from build123d import *

# Parameters (mm, degrees)
SKETCH_2_W          = 40
SKETCH_2_H          = 57
CUT_EXTRUDE_1_DEPTH = 4
SKETCH_3_R          = 7
CUT_EXTRUDE_3_DEPTH = 4


with BuildPart() as part:
    # 草圖1 → 旋轉1 (revolve)
    with BuildSketch(Plane.XY):
        Polygon((0, 21), (25, 21), (25, 0), (28.5, 0), (28.5, -2), (12.5, -2), (12.5, -21.7), (8, -21.7), (8, 2.3), (0, 2.3), align=None)
    revolve(axis=Axis((0, 41.921070153, 0), (0, -1, 0)))

    # 草圖2 → 除料-伸長1 (cut)
    with BuildSketch(Plane(origin=(0, 21, 0), x_dir=(1, 0, 0), z_dir=(0, 1, 0))):
        Rectangle(SKETCH_2_W, SKETCH_2_H)
    extrude(amount=-CUT_EXTRUDE_1_DEPTH, mode=Mode.SUBTRACT)

    # 草圖3 → 除料-伸長3 (cut)
    with BuildSketch(Plane(origin=(0, 17, 0), x_dir=(1, 0, 0), z_dir=(0, 1, 0))):
        Circle(SKETCH_3_R)
    extrude(amount=-CUT_EXTRUDE_3_DEPTH, mode=Mode.SUBTRACT)


solid = part.part
Source: CAD feature listing. Evaluate the final solid. Frame: model axes, mm. A direction names the side the tool comes from. Round coordinates to 2 decimals unless told otherwise and drop trailing zeros. Loops run counter-clockwise (first coordinate to the right, second up) from the corner with the lowest first, then second, coordinate; pieces in that order, holes last.
Q1. Section A-A, the plane x = 0. Return loops of the section in (y, z), plus the area to 3 significant figures.
Q2. Ray query, line 1 (X direction, y = 14.7, z = 0); line 2 (Y direction, x = -8.5, z = 22.5). Return the intervals inside material, ascending.
Q3. First-contact query: P1, Ø4, axis at x = -13.5, y = -1, coming from the -Z side; P2, Ø1, axis at x = 13, y = 2.5, coming from the +Z side; P3, Ø15.5, axis at x = -1, z = 2, coming from the +Y side; P4, Ø6, axis at x = -1.5, z = 7, coming from the -Y side. Flat tips, straight axial feed; report the tip coordinate or a pass-through.
Q4. Section D-D, the plane z = 0. Return loops of the section in (x, y), plus the area to 3 significant figures.
Q5. Section B-B, the plane z = 21.5. Return loops of the section in (x, y).
Q6. Access query for faces 1 (the face through (-22, 21, 0)), 2 (the face through (26.327, -1.014, -10.916)), 3 (the face through (-1.73, -9.53, -7.81)), 4 (the face through (6.466, 15.028, 2.681)), 5 (the face through (-5, 17, -6)). Directions: +Z, -Z, +X, -X, +Y, -Y. A direction counts if a zero-diameter tool reaches every point of the face in a straight line with its end or side. Return the directions, or none.
Q7. Mould query, pull axis Z, two halves, no side actions, for faces 6 (the face through (-0.2, -21.7, -8.2)), 7 (the face through (0, 13, 0)), 8 (the face through (11.923, -11.988, 3.755)). Classes: pulls with the +Z half, pulls with the -Z half, needs draft (parallel to the pull), parting line crosses it, or undercut.
Q8. Section C-C, the plane y = 1.5. Return loops of the section in (x, z).
Solutions:
1. outline: (-21.7, -12.5) - (-2, -12.5) - (-2, -28.5) - (0, -28.5) - (0, -25) - (17, -25) - (17, -7) - (13, -7) - (13, 7) - (17, 7) - (17, 25) - (0, 25) - (0, 28.5) - (-2, 28.5) - (-2, 12.5) - (-21.7, 12.5) - (-21.7, 8) - (2.3, 8) - (2.3, -8) - (-21.7, -8) - close
1. area: 1,020 mm2
2. line 1: x = -25 to -7, 7 to 25
2. line 2: y = -2 to 17
3. P1: stops at z = -26.08
3. P2: stops at z = 21.65
3. P3: stops at y = 17
3. P4: stops at y = -21.7
4. outline: (-28.5, -2) - (-12.5, -2) - (-12.5, -21.7) - (-8, -21.7) - (-8, 2.3) - (8, 2.3) - (8, -21.7) - (12.5, -21.7) - (12.5, -2) - (28.5, -2) - (28.5, 0) - (25, 0) - (25, 21) - (20, 21) - (20, 17) - (7, 17) - (7, 13) - (-7, 13) - (-7, 17) - (-20, 17) - (-20, 21) - (-25, 21) - (-25, 0) - (-28.5, 0) - close
4. area: 1,060 mm2
5. outline: (-18.71, -2) - (18.71, -2) - (18.71, 0) - (12.76, 0) - (12.76, 17) - (-12.76, 17) - (-12.76, 0) - (-18.71, 0) - close
6. face 1: +Z, -Z, +X, -X, +Y
6. face 2: +Y, -Y
6. face 3: -Y
6. face 4: +Y
6. face 5: +Z, -Z, +Y
7. face 6: needs draft
7. face 7: undercut
7. face 8: parting line crosses it
8. outline: circle Ø50 at (0, 0); hole circle Ø16 at (0, 0)
